Design review of the part built by this model. Coordinates are the model's own, in mm. A direction names the side the tool comes from. Coordinates: 2 decimals unless noted, no trailing zeros. Write each loop counter-clockwise with the first axis right and the second up, starting at its lowest first coordinate (ties: lowest second). Pieces come first, ordered by that corner, then holes. Notation, with made-up numbers: (41, -28.5) - (94, -28.5) arc R13 ccw to (94, -11.5) - close; hole circle Ø6 at (18, -37.5). An arc over 180 degrees is marked (long way). Use a Markdown table: item, result.
from build123d import *

# Parameters (mm, degrees)
SKETCH1_R           = 9
SKETCH1_R_2         = 3
SKETCH1_R_3         = 5
BOSS_EXTRUDE1_DEPTH = 10
SKETCH_L_R          = 6
BOSS_EXTRUDE2_DEPTH = 4
SKETCH6_R           = 4
BOSS_EXTRUDE3_DEPTH = 4


with BuildPart() as part:
    # Sketch1 → Boss-Extrude1 (new body)
    with BuildSketch(Plane(origin=(0, 0, 0), x_dir=(1, 0, 0), z_dir=(0, 1, 0))):
        with BuildLine():
            Line((5.562305899, -17.119017293), (93.090169944, 11.320509704))
            ThreePointArc((93.090169944, 11.320509704), (99.876883406, 22.395419517), (90, 30.831074867))
            Line((90, 30.831074867), (12.860666935, 30.831074867))
            ThreePointArc((12.860666935, 30.831074867), (4.846689129, 31.602733162), (-2.872809988, 33.889352975))
            Line((-2.872809988, 33.889352975), (-45.75236044, 51.21381591))
            ThreePointArc((-45.75236044, 51.21381591), (-52.728064522, 49.344681634), (-52.854101966, 42.124001268))
            Line((-52.854101966, 42.124001268), (-14.562305899, -10.580134541))
            ThreePointArc((-14.562305899, -10.580134541), (-5.562305899, -17.119017293), (5.562305899, -17.119017293))
        make_face()
        with Locations(Location((0, 0, 0), (0, 0, 270))):
            Circle(SKETCH1_R, mode=Mode.SUBTRACT)
        with Locations(Location((-48, 45.650712782, 0), (0, 0, 270))):
            Circle(SKETCH1_R_2, mode=Mode.SUBTRACT)
        with Locations(Location((90, 20.831074867, 0), (0, 0, 270))):
            Circle(SKETCH1_R_3, mode=Mode.SUBTRACT)
    extrude(amount=BOSS_EXTRUDE1_DEPTH)

    # Sketch l → Boss-Extrude2 (add)
    with BuildSketch(Plane(origin=(32.335921554, 0, -10.506577809), x_dir=(0, -1, 0), z_dir=(-0.9510565162951555, 0, 0.3090169943749418))):
        with BuildLine():
            Line((-10, 18), (-58, 18))
            ThreePointArc((-58, 18), (-69.934262744, 7.254341559), (-60.49494029, -5.737771209))
            Line((-60.49494029, -5.737771209), (-10, -16.470802099))
            Line((-10, -16.470802099), (-10, 18))
        make_face()
        with Locations(Location((-58, 6, 0), (0, 0, 90))):
            Circle(SKETCH_L_R, mode=Mode.SUBTRACT)
    extrude(amount=-BOSS_EXTRUDE2_DEPTH)

    # Sketch6 → Boss-Extrude3 (add)
    with BuildSketch(Plane(origin=(-19.984698578, 0, -27.506577809), x_dir=(0, -1, 0), z_dir=(-0.5877852522924776, 0, -0.8090169943749442))):
        with BuildLine():
            Line((-10, 18), (-56, 18))
            ThreePointArc((-56, 18), (-63.92214455, 11.113384808), (-58.205098847, 2.309906432))
            Line((-58.205098847, 2.309906432), (-10, -11.512683232))
            Line((-10, -11.512683232), (-10, 18))
        make_face()
        with Locations(Location((-56, 10, 0), (0, 0, 90))):
            Circle(SKETCH6_R, mode=Mode.SUBTRACT)
    extrude(amount=BOSS_EXTRUDE3_DEPTH)


solid = part.part
(1) Take a section at B-B on x = -48. Write out the cut boundary in (y, z).
Determined:
| item | result |
|---|---|
| outline | (0, -51.65) - (10, -51.65) - (10, -48.65) - (0, -48.65) - close; (0, -42.65) - (10, -42.65) - (10, -35.44) - (0, -35.44) - close |
(2) Take a section at C-C on y = 5.5. Write out the cut boundary in (x, z), and give its area (3 significant figures).
Determined:
| item | result |
|---|---|
| outline | (-52.85, -42.12) arc R6 ccw to (-45.75, -51.21) - (-2.87, -33.89) arc R42 cw to (12.86, -30.83) - (90, -30.83) arc R10 ccw to (93.09, -11.32) - (5.56, 17.12) arc R18 ccw to (-14.56, 10.58) - close; hole circle Ø6 at (-48, -45.65); hole circle Ø18 at (0, 0); hole circle Ø10 at (90, -20.83) |
| area | 4,880 mm2 |
(3) Machinability: for faces 1 (the cylindrical face through (99.906, 4.93, -22.2)), 2 (the flat face through (30.803, 35.601, -21.605)), 3 (the flat face through (52, 5, -30.831)), 4 (the flat face through (37.635, 33.753, -7.143)), which of the approach directions +Z, -Z, +X, -X, +Y, -Y give a long, thin tool a straight path to every point of the face, cutting with its end or side? Answer none if there is none.
Determined:
| item | result |
|---|---|
| face 1 | +X, +Y, -Y |
| face 2 | -Z, +Y |
| face 3 | -Z, +X, +Y, -Y |
| face 4 | -Z, +X, +Y |
(4) For L1, parallel to Y at x = 11.5, z = -13.5; L2, parallel to X at y = 7, z = -22; L3, parallel to X at y = 14.5, z = -24, list the stretches that pass through material, from the lowest coordinate up. Write a range as from..to.
Determined:
| item | result |
|---|---|
| L1 | 0..10 |
| L2 | -38.23..85.14, 94.86..99.93 |
| L3 | -31.62..-24.81, 27.95..32.16 |
(5) For pin 1 (1.5 mm diameter, centred on y = 12.5, z = -29, fed in from +X); pin 2 (2 mm diameter, centred on x = -0.5, z = 10.5, fed in from +Y); pin 3 (11 mm diameter, centred on x = 53.5, y = 4.5, fed in from -Z), all flat-tipped, find the tip position at first contact; note any pin that passes through.
Determined:
| item | result |
|---|---|
| pin 1 | x = -16.9 |
| pin 2 | y = 10 |
| pin 3 | z = -30.83 |
(6) Take a section at A-A on y = 40. Write out the cut boundary in (x, z).
Determined:
| item | result |
|---|---|
| outline | (-36.9, -20.16) - (-19.98, -32.45) - (-17.63, -29.22) - (-34.55, -16.93) - close; (29.22, -20.11) - (33.02, -21.34) - (41.7, 5.38) - (37.9, 6.61) - close |
(7) Take a section at D-D on z = -39. Write out the cut boundary in (x, y), and give its area (3 significant figures).
Determined:
| item | result |
|---|---|
| outline | (-50.58, 0) - (-15.52, 0) - (-15.52, 10) - (-50.58, 10) - close |
| area | 351 mm2 |
(8) Draft analysis for pull direction X (two halves, no side actions). For faces 5 (the flat face through (-24.01, 4.93, -42.43)), 6 (the cylindrical face through (-28.532, 52.095, -23.734)), 7 (the cylindrical face through (-5.71, 4.93, 17.07)), 8 (the flat face through (22, 10, -17)), state which applies: +X half, -X half, draft (parallel to the pull), parting line (faces both ways), or undercut.
Determined:
| item | result |
|---|---|
| face 5 | +X half |
| face 6 | undercut |
| face 7 | parting line |
| face 8 | undercut |
